```python
from build123d import *

# Parameters (mm, degrees)
F0_W     = 10
F0_H     = 15
F1_DEPTH = 10
F4_R     = 0.5


with BuildPart() as f1:
    # F0 (on Top) → F1 (new body)
    with BuildSketch(Plane.XY):
        Rectangle(F0_W, F0_H)
    extrude(amount=-F1_DEPTH)

    # F2 (on face) → F3 (revolve, cut)
    with BuildSketch(Plane.XY):
        with BuildLine():
            ThreePointArc((1.8027756377, 0), (3.3726843908, 3.9354143467), (0, 6.5))
            Line((0, 6.5), (0, 0.5))
            ThreePointArc((0, 0.5), (0.9354143467, 0.3726843908), (1.8027756377, 0))
        make_face()
        with BuildLine():
            ThreePointArc((1.8027756377, 0), (0.9354143467, 0.3726843908), (0, 0.5))
            Line((0, 0.5), (0, -0.5))
            ThreePointArc((0, -0.5), (0.9354143467, -0.3726843908), (1.8027756377, 0))
        make_face()
        with BuildLine():
            ThreePointArc((0, -6.5), (3.3726843908, -3.9354143467), (1.8027756377, 0))
            ThreePointArc((1.8027756377, 0), (0.9354143467, -0.3726843908), (0, -0.5))
            Line((0, -0.5), (0, -6.5))
        make_face()
    revolve(axis=Axis((0, 0.2168327096, 0), (0, -1, 0)), mode=Mode.SUBTRACT)

    # F4
    f4_edges = [f1.edges().sort_by_distance(p)[0] for p in [
        (3.372684, 3.935414, 0),
        (-3.372684, 3.935414, 0),
        (3.372684, -3.935414, 0),
        (-3.372684, -3.935414, 0),
    ]]
    fillet(f4_edges, radius=F4_R)


solid = f1.part
```
Build history of the part. All positions in model axes, mm. Coordinates: 2 decimals unless noted, no trailing zeros. Order: outer loops, then holes, each group sorted by start corner. A loop starts at its lowest first (then second) coordinate and runs counter-clockwise, first axis right, second up. Notation, with made-up numbers: (45.5, 68.5) -> (51.5, 68.5) arc R15 cw to (51.5, 75.5) -> close; hole circle Ø6 at (36.5, 28). An arc over 180 degrees is marked (long way). Answer in a Markdown table with one row per item. Add a question column.
Q1. Band-saw the part on B-B, the plane z = -2.5. List the corners of the cut face in (x, y), then the cut area to 3 significant figures.
Q2. Wall check: line 1 along X through (y, z) = (-4, -2.5); line 2 along X through (y, z) = (1.5, -2); line 3 along Z through (x, y) = (2.5, 5). Give the ranges that are in metal, low to high. Write a range as [from, to].
Q3. Band-saw the part on A-A, the plane z = -1. List the corners of the cut face in (x, y).
Q4. Drop a flat-ended pin along its axis: pin 1 (1 mm diameter, centred on x = 1, y = 0, fed in from +Z). Give the stop position or say it passes through.
Answers follow:
| question | item | result |
|---|---|---|
| 1 | outline | (-5, -7.5) -> (5, -7.5) -> (5, 7.5) -> (-5, 7.5) -> close; hole circle Ø4.9 at (0, -3); hole circle Ø4.9 at (0, 3) |
| 1 | area | 112 mm^2 |
| 2 | line 1 | [-5, -2.24], [2.24, 5] |
| 2 | line 2 | [-5, -2.45], [2.45, 5] |
| 2 | line 3 | [-10, -1.41] |
| 3 | outline | (-5, -7.5) -> (5, -7.5) -> (5, 7.5) -> (-5, 7.5) -> close; hole (-1.5, 0) arc R3.35 ccw (long way) to (1.5, 0) arc R3.35 ccw (long way) to start |
| 4 | pin 1 | z = -1 |
